The listing builds one solid part. Answer for the finished solid, in the listing's coordinates (mm). Coordinates: 2 decimals unless noted, no trailing zeros. Write each loop counter-clockwise with the first axis right and the second up, starting at its lowest first coordinate (ties: lowest second). Pieces come first, ordered by that corner, then holes. Notation, with made-up numbers: M 27,80.25 L 52,80.25 A22 cw 52,106.25 Z; hole C 34.5,29.25 d4. An arc over 180 degrees is marked long. Answer as a JSON object with one key per item and string values. Group by question number.
from build123d import *

# Parameters (mm, degrees)
SKETCH1_W               = 19
SKETCH1_H               = 19
SKETCH1_W_2             = 17
SKETCH1_H_2             = 17
BOSS_EXTRUDE1_DEPTH     = 400
CUT_EXTRUDE3_DEPTH      = 1
CUT_EXTRUDE3_DEPTH_BACK = 20
CUT_EXTRUDE4_DEPTH      = 1
CUT_EXTRUDE4_DEPTH_BACK = 20


with BuildPart() as part:
    # Sketch1 → Boss-Extrude1 (new body)
    with BuildSketch(Plane.XY):
        Rectangle(SKETCH1_W, SKETCH1_H)
        Rectangle(SKETCH1_W_2, SKETCH1_H_2, mode=Mode.SUBTRACT)
    extrude(amount=BOSS_EXTRUDE1_DEPTH)

    # Sketch2 → Cut-Extrude3 (cut, two sides)
    with BuildSketch(Plane.XZ.offset(9.5)) as cut_extrude3_sk:
        Polygon((-711.761724625, -405.450995754), (-9.5, 0), (9.5, 10.969655115), (711.761724625, 416.420650868), (1522.663716132, -988.102798381), (99.140266883, -1809.974445003), align=None)
    extrude(amount=CUT_EXTRUDE3_DEPTH, mode=Mode.SUBTRACT)
    extrude(cut_extrude3_sk.sketch, amount=-CUT_EXTRUDE3_DEPTH_BACK, mode=Mode.SUBTRACT)

    # Sketch3 → Cut-Extrude4 (cut, two sides)
    with BuildSketch(Plane(origin=(0, -9.5, 0), x_dir=(-1, 0, 0), z_dir=(0, -1, 0))) as cut_extrude4_sk:
        Polygon((711.761724625, -805.450995754), (9.5, -400), (-9.5, -389.030344885), (-711.761724625, 16.420650868), (-1522.663716132, -1388.102798381), (-99.140266883, -2209.974445003), align=None)
    extrude(amount=CUT_EXTRUDE4_DEPTH, mode=Mode.SUBTRACT)
    extrude(cut_extrude4_sk.sketch, amount=-CUT_EXTRUDE4_DEPTH_BACK, mode=Mode.SUBTRACT)


solid = part.part
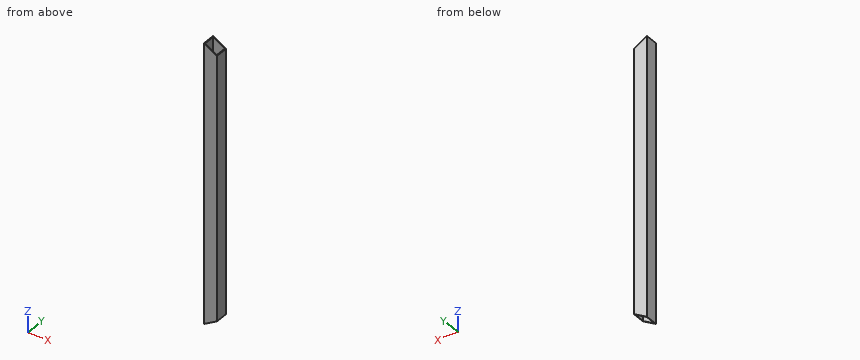
Item 1: Consider L1, parallel to X at y = -5, z = 58.5; L2, parallel to Z at x = 8.75, y = -8. Determine where each line is inside the solid, lowest interval first. Write a range as from..to.
Item 2: A cutting plane is placed at C-C, the plane x = -5. Write down the section's boundary in (y, z), and give its area (3 significant figures).
Item 3: A cutting plane is placed at B-B, the plane z = 77. Write down the section's boundary in (x, y).
Item 4: Flat-ended cylindrical pins translate along their axes: pin 1 Ø6 at (x, y) = (5, 7.5) entering from -Z; pin 2 Ø4 at (x, y) = (7, 2.5) entering from -Z. Find the tip coordinate at first contact, or state that the pin passes through.
Item 5: A cutting plane is placed at A-A, the plane y = 0.5. Write down the section's boundary in (x, z).
Answer:
{
 "1": {"L1": "-9.5..-8.5, 8.5..9.5", "L2": "10.54..389.46"},
 "2": {"outline": "M -9.5,2.6 L -8.5,2.6 L -8.5,397.4 L -9.5,397.4 Z; M 8.5,2.6 L 9.5,2.6 L 9.5,397.4 L 8.5,397.4 Z", "area": "790 mm2"},
 "3": {"outline": "M -9.5,-9.5 L 9.5,-9.5 L 9.5,9.5 L -9.5,9.5 Z; hole M -8.5,-8.5 L 8.5,-8.5 L 8.5,8.5 L -8.5,8.5 Z"},
 "4": {"pin 1": "z = 6.74", "pin 2": "z = 10.39"},
 "5": {"outline": "M -9.5,0 L -8.5,0.58 L -8.5,399.42 L -9.5,400 Z; M 8.5,10.39 L 9.5,10.97 L 9.5,389.03 L 8.5,389.61 Z"}
}
